Verification items for this drawing (mm, ordinates from the low corner). A direction names the side the tool comes from. Give positions to 0.01 mm unless a question says otherwise; leave off trailing zeros. Loops run counter-clockwise (first coordinate to the right, second up) from the corner with the lowest first, then second, coordinate; pieces in that order, holes last. Notation, with made-up numbers: M 18,15 L 28,15 A13 cw 28,19 Z; hole C 72,15.25 d9. An arc over 180 degrees is marked long. Use one line per item in the form item = value.
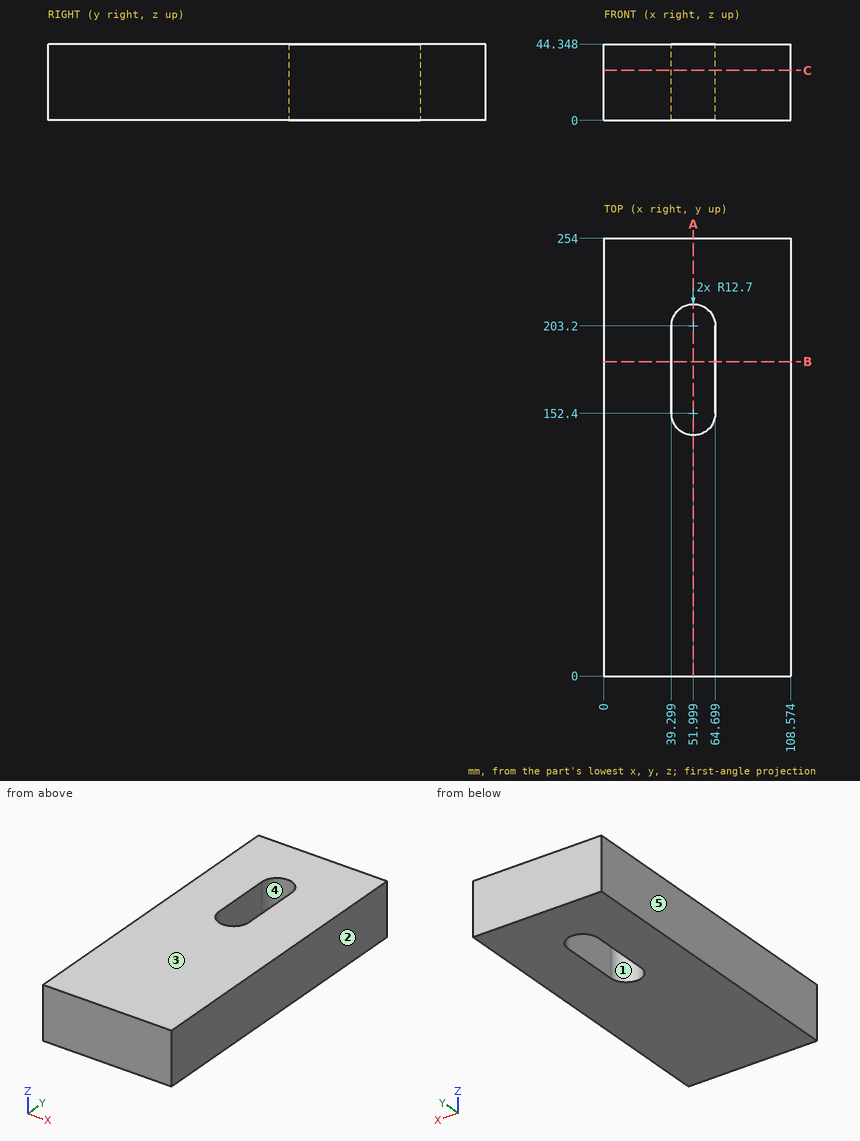
1) Section check B-B (y = 182.5). Record the cut outline in (x, z).
Evaluation:
outline = M 0,0 L 39.3,0 L 39.3,44.35 L 0,44.35 Z; M 64.7,0 L 108.57,0 L 108.57,44.35 L 64.7,44.35 Z
2) Section check A-A (x = 52). Record the cut outline in (y, z).
Evaluation:
outline = M 0,0 L 139.7,0 L 139.7,44.35 L 0,44.35 Z; M 215.9,0 L 254,0 L 254,44.35 L 215.9,44.35 Z
3) Scan lines: line 1 (X direction, y = 176.5, z = 9); line 2 (Y direction, x = 59.5, z = 23.5); line 3 (X direction, y = 144, z = 9.5) (1 decimal). Record each from-to range of solid material in increasing order.
Evaluation:
line_1 = 0 to 39.3, 64.7 to 108.57
line_2 = 0 to 142.15, 213.45 to 254
line_3 = 0 to 42.5, 61.5 to 108.6
4) Release check for a two-part mould opening along X. For the marked faces 1, 2 and 3 record: pulls with the +X half, pulls with the -X half, needs draft (parallel to the pull), parting line crosses it, or undercut.
Evaluation:
face_1 = undercut
face_2 = pulls with the +X half
face_3 = needs draft
5) Set-up check for the marked faces 4 and 5: record each of +Z, -Z, +X, -X, +Y, -Y from which the full face is reachable in a straight line by a thin tool's end or side.
Evaluation:
face_4 = +Z, -Z
face_5 = +Z, -Z, -X, +Y, -Y
6) Section check C-C (z = 29). Record the cut outline in (x, y), then the cut area to 3 significant figures.
Evaluation:
outline = M 0,0 L 108.57,0 L 108.57,254 L 0,254 Z; hole M 39.3,152.4 A12.7 ccw 64.7,152.4 L 64.7,203.2 A12.7 ccw 39.3,203.2 Z
area = 25,800 mm^2
